Autodesk Inventor part; units mm, degrees
ref_plane "YZ Plane" through (0, 0, 0) normal (1, 0, 0) x (0, 1, 0)
ref_plane "XZ Plane" through (0, 0, 0) normal (0, 1, 0) x (-1, 0, 0)
ref_plane "XY Plane" through (0, 0, 0) normal (0, 0, 1) x (1, 0, 0)
sketch "Sketch1" plane through (0, 0, 0) normal (0, 1, 0) x (-1, 0, 0)
  line L0 (-21, -21) -> (21, -21)
  line L1 (21, -21) -> (21, 21)
  line L2 (21, 21) -> (-21, 21)
  line L3 (-21, 21) -> (-21, -21)
  line L4 (-21, -21) -> (21, 21) construction
  line L5 (21, -21) -> (-21, 21) construction
  circle A0 centre (15.5, 15.5) radius 1.75
  circle A1 centre (0, 0) radius 10.75
  line L6 (34.796, 0) -> (-29.6686, 0)
  line L7 (0, -38.1967) -> (0, 38.2612)
  circle A2 centre (15.5, -15.5) radius 1.75
  circle A3 centre (-15.5, 15.5) radius 1.75
  circle A4 centre (-15.5, -15.5) radius 1.75
  dimension "d0" = 42
  dimension "d1" = 42
  dimension "d4" = 3.5
  dimension "d8" = 21.5
  dimension "d13" = 31
extrude "Extrusion4" add sketch "Sketch1" along normal blind 4.7625 contours L3 L6 A1 L7 L0 | L7 A1 L6 L1 L0 | L3 L2 L7 A1 L6 | L6 A1 L7 L2 L1
equation "\"d0\" = d1"
properties part number "Vertical_Lead_Screw_Shaft_Mount_Plate_End"
Read the model definition and answer for the solid it produces. Units are mm, in the model's axes. Coordinates: 2 decimals unless noted, no trailing zeros. Loops run counter-clockwise (first coordinate to the right, second up) from the corner with the lowest first, then second, coordinate; pieces in that order, holes last. Notation, with made-up numbers: (23.5, 81) -> (59.5, 81) arc R14 cw to (59.5, 103) -> close; hole circle Ø10 at (52, 33). An arc over 180 degrees is marked (long way). Return JSON: item names as keys, results as strings.
Item 1: Find section A-A (z = 15.5). Determine the outline of the cut face in (x, y).
Answers:
{"outline": "(-21, 0) -> (-17.25, 0) -> (-17.25, 4.76) -> (-21, 4.76) -> close; (-13.75, 0) -> (13.75, 0) -> (13.75, 4.76) -> (-13.75, 4.76) -> close; (17.25, 0) -> (21, 0) -> (21, 4.76) -> (17.25, 4.76) -> close"}
Item 2: Find section B-B (y = 3.7). Determine the outline of the cut face in (x, z).
Answers:
{"outline": "(-21, -21) -> (21, -21) -> (21, 21) -> (-21, 21) -> close; hole circle Ø3.5 at (-15.5, -15.5); hole circle Ø3.5 at (-15.5, 15.5); hole circle Ø21.5 at (0, 0); hole circle Ø3.5 at (15.5, -15.5); hole circle Ø3.5 at (15.5, 15.5)"}
Item 3: Find section C-C (x = 0). Determine the outline of the cut face in (y, z), plus the area to 3 significant figures.
Answers:
{"outline": "(0, -21) -> (4.76, -21) -> (4.76, -10.75) -> (0, -10.75) -> close; (0, 10.75) -> (4.76, 10.75) -> (4.76, 21) -> (0, 21) -> close", "area": "97.6 mm2"}
Item 4: Find section D-D (x = -15.5). Determine the outline of the cut face in (y, z), plus the area to 3 significant figures.
Answers:
{"outline": "(0, -21) -> (4.76, -21) -> (4.76, -17.25) -> (0, -17.25) -> close; (0, -13.75) -> (4.76, -13.75) -> (4.76, 13.75) -> (0, 13.75) -> close; (0, 17.25) -> (4.76, 17.25) -> (4.76, 21) -> (0, 21) -> close", "area": "167 mm2"}
Item 5: Find the intervals of material crossed by probe 1 along Z at (x, y) = (-15.5, 3.4); probe 2 along Z at (x, y) = (14.5, 0.5), in increasing order.
Answers:
{"probe 1": "z = -21 to -17.25, -13.75 to 13.75, 17.25 to 21", "probe 2": "z = -21 to -16.94, -14.06 to 14.06, 16.94 to 21"}
Item 6: For a pull along Z with two mould halves and no side action, classify faces 1 (the flat face through (5, 0, 10)), 2 (the cylindrical face through (14.6, 2.3, -17)), 3 (the flat face through (0, 2, -21)), 4 (the flat face through (0, 2, 21)) as +Z half, -Z half, draft (parallel to the pull), parting line (faces both ways), or undercut.
Answers:
{"face 1": "draft", "face 2": "undercut", "face 3": "-Z half", "face 4": "+Z half"}
